Verification items for the finished model (mm, model axes). A direction names the side the tool comes from. Give positions to 0.01 mm unless a question says otherwise; leave off trailing zeros. Loops run counter-clockwise (first coordinate to the right, second up) from the corner with the lowest first, then second, coordinate; pieces in that order, holes last. Notation, with made-up numbers: (17, -12.75) - (59, -12.75) arc R30 ccw to (59, 10.25) - close; hole circle Ø7 at (-33, 62.25). An arc over 180 degrees is marked (long way). Answer in a Markdown table with one row per item.
```python
from build123d import *

# Parameters (mm, degrees)
EXTRUDE_1_DEPTH     = 3
SKETCH_4_W          = 13
SKETCH_4_H          = 8
EXTRUDE_2_DEPTH     = 7
EXTRUDE_6_DEPTH     = 20
CUT_EXTRUDE_3_DEPTH = 34.531337759
EXTRUDE_7_DEPTH     = 16
SKETCH_18_W         = 6.2
SKETCH_18_H         = 1
CUT_EXTRUDE_6_DEPTH = 20
SKETCH_19_R         = 1
CUT_EXTRUDE_7_DEPTH = 3
EXTRUDE_8_DEPTH     = 12
SKETCH_24_W         = 2.5
SKETCH_24_H         = 9.5
CUT_EXTRUDE_8_DEPTH = 20
SKETCH_25_W         = 5
SKETCH_25_H         = 5.2
CUT_EXTRUDE_9_DEPTH = 1


with BuildPart() as part:
    # 草图1 → 凸台-拉伸1 (new body)
    with BuildSketch(Plane(origin=(0, 0, 0), x_dir=(1, 0, 0), z_dir=(0, 1, 0))):
        Polygon((24, 0), (12, 20.784609691), (-12, 20.784609691), (-24, 0), (-12, -20.784609691), (12, -20.784609691), align=None)
    extrude(amount=EXTRUDE_1_DEPTH)

    # 草图4 → 凸台-拉伸2 (add)
    with BuildSketch(Plane(origin=(0, 3, 0), x_dir=(1, 0, 0), z_dir=(0, 1, 0))):
        with Locations((0, -8.746728068)):
            Rectangle(SKETCH_4_W, SKETCH_4_H)
    extrude(amount=EXTRUDE_2_DEPTH)

    # 草图14 → 凸台-拉伸6 (add)
    with BuildSketch(Plane.XY.offset(12.746728068)):
        with BuildLine():
            Line((-6.5, 10), (-6.5, 6.5))
            ThreePointArc((-6.5, 6.5), (0, 5.267826192), (6.5, 6.5))
            Line((6.5, 6.5), (6.5, 10))
            ThreePointArc((6.5, 10), (0, 8.436464997), (-6.5, 10))
        make_face()
    extrude(amount=EXTRUDE_6_DEPTH)

    # 草图15 → 切除-拉伸3 (cut, through all)
    with BuildSketch(Plane.XY.offset(12.746728068)):
        with BuildLine():
            Line((6.5, 10), (-6.5, 10))
            ThreePointArc((-6.5, 10), (0, 8.436464997), (6.5, 10))
        make_face()
    extrude(amount=-CUT_EXTRUDE_3_DEPTH, mode=Mode.SUBTRACT)

    # 草图16 → 凸台-拉伸7 (add)
    with BuildSketch(Plane(origin=(0, 3, 0), x_dir=(1, 0, 0), z_dir=(0, 1, 0))):
        with BuildLine():
            Line((6.5, 13.284609691), (6.5, 11.284609691))
            ThreePointArc((6.5, 11.284609691), (0, 12.623387741), (-6.5, 11.284609691))
            Line((-6.5, 11.284609691), (-6.5, 13.284609691))
            ThreePointArc((-6.5, 13.284609691), (0, 14.747919911), (6.5, 13.284609691))
        make_face()
    extrude(amount=EXTRUDE_7_DEPTH)

    # 草图18 → 切除-拉伸6 (cut, through all)
    with BuildSketch(Plane.XZ):
        Polygon((10.319872981, 13.694675051), (9.453847577, 13.194675051), (12.553847577, 7.825317547), (13.419872981, 8.325317547), align=None)
        Polygon((13.053847577, 6.959292144), (13.919872981, 7.459292144), (17.019872981, 2.08993464), (16.153847577, 1.58993464), align=None)
        with Locations((3.6, -15.284609691)):
            Rectangle(SKETCH_18_W, SKETCH_18_H)
        with Locations((-3.6, -15.284609691)):
            Rectangle(SKETCH_18_W, SKETCH_18_H)
        Polygon((-16.153847577, 1.58993464), (-13.053847577, 6.959292144), (-13.919872981, 7.459292144), (-17.019872981, 2.08993464), align=None)
        Polygon((-12.553847577, 7.825317547), (-13.419872981, 8.325317547), (-10.319872981, 13.694675051), (-9.453847577, 13.194675051), align=None)
    extrude(amount=-CUT_EXTRUDE_6_DEPTH, mode=Mode.SUBTRACT)

    # 草图19 → 切除-拉伸7 (cut)
    with BuildSketch(Plane.XZ):
        with Locations((0, 17.784609691)):
            Circle(SKETCH_19_R)
        with Locations((15.401923789, -8.892304845)):
            Circle(SKETCH_19_R)
        with Locations((-15.401923789, -8.892304845)):
            Circle(SKETCH_19_R)
    extrude(amount=-CUT_EXTRUDE_7_DEPTH, mode=Mode.SUBTRACT)

    # 草图23 → 凸台-拉伸8 (add)
    with BuildSketch(Plane.XY.offset(32.746728068)):
        with BuildLine():
            Line((-9.532090727, 12.079217693), (-9.532090727, 8.042497168))
            ThreePointArc((-9.532090727, 8.042497168), (0, 5.267826192), (9.532090727, 8.042497168))
            Line((9.532090727, 8.042497168), (9.532090727, 12.079217693))
            ThreePointArc((9.532090727, 12.079217693), (0, 8.436464997), (-9.532090727, 12.079217693))
        make_face()
    extrude(amount=EXTRUDE_8_DEPTH)

    # 草图24 → 切除-拉伸8 (cut, through all)
    with BuildSketch(Plane.XZ):
        with Locations((-7.282090727, 38.496728068)):
            Rectangle(SKETCH_24_W, SKETCH_24_H)
        with Locations((7.282090727, 38.496728068)):
            Rectangle(SKETCH_24_W, SKETCH_24_H)
    extrude(amount=-CUT_EXTRUDE_8_DEPTH, mode=Mode.SUBTRACT)

    # 草图25 → 切除-拉伸9 (cut)
    with BuildSketch(Plane.XZ):
        Polygon((-10.532695155, -0.673943767), (-6.029363055, -3.273943767), (-3.529363055, 1.056183252), (-8.032695155, 3.656183252), align=None)
        Polygon((-7.182695155, 5.128426439), (-4.682695155, 9.458553458), (-0.179363055, 6.858553458), (-2.679363055, 2.528426439), align=None)
        Polygon((6.029363055, -3.273943767), (3.529363055, 1.056183252), (8.032695155, 3.656183252), (10.532695155, -0.673943767), align=None)
        Polygon((0.179363055, 6.858553458), (2.679363055, 2.528426439), (7.182695155, 5.128426439), (4.682695155, 9.458553458), align=None)
        with Locations((-3.35, -6.184609691)):
            Rectangle(SKETCH_25_W, SKETCH_25_H)
        with Locations((3.35, -6.184609691)):
            Rectangle(SKETCH_25_W, SKETCH_25_H)
    extrude(amount=-CUT_EXTRUDE_9_DEPTH, mode=Mode.SUBTRACT)


solid = part.part
```
Q1. Thickness scan on line 1 (X direction, y = 10.75, z = 38.5); line 2 (Y direction, x = 18, z = -4); line 3 (X direction, y = 11.75, z = 39). Record the ranges inside material, lowest first.
Completed:
| item | result |
|---|---|
| line 1 | -9.53 to -8.53, 8.53 to 9.53 |
| line 2 | 0 to 3 |
| line 3 | -9.53 to -9.15, 9.15 to 9.53 |
Q2. Sectioned sample at D-D (z = 32). Record the cut outline in (x, y), and give its area (3 significant figures).
Completed:
| item | result |
|---|---|
| outline | (-6.5, 6.5) arc R17.76 ccw to (6.5, 6.5) - (6.5, 10) arc R14.29 cw to (-6.5, 10) - close |
| area | 42.5 mm^2 |
Q3. Draft check along X on faces 1 (the face through (-6.5, 11, -12)), 2 (the face through (14.66, 1.48, -8.22)), 3 (the face through (0, 1, 20.785)). Enter one of: +X half, -X half, draft (parallel to the pull), parting line (faces both ways), or undercut.
Completed:
| item | result |
|---|---|
| face 1 | -X half |
| face 2 | undercut |
| face 3 | draft |
Q4. Sectioned sample at C-C (y = 17.75). Record the cut outline in (x, z), and give its area (3 significant figures).
Completed:
| item | result |
|---|---|
| outline | (-6.5, -13.28) arc R15.17 ccw to (6.5, -13.28) - (6.5, -11.28) arc R16.45 cw to (-6.5, -11.28) - close |
| area | 27.1 mm^2 |
Q5. Go/stop test with flat-tipped pins: P1, Ø4, axis at y = 10.5, z = 11.5, coming from the -X side; P2, Ø2.5, axis at x = 2.5, z = -7, coming from the -Y side; P3, Ø0.5, axis at y = 0.5, z = -5, coming from the -X side. Record where each tip stops, or that it passes through.
Completed:
| item | result |
|---|---|
| P1 | x = -6.5 |
| P2 | y = 1 |
| P3 | x = -21.26 |
Q6. Sectioned sample at B-B (x = 2). Record the cut outline in (y, z), and give its area (3 significant figures).
Completed:
| item | result |
|---|---|
| outline | (0, -20.78) - (3, -20.78) - (3, -15.78) - (0, -15.78) - close; (0, -14.78) - (3, -14.78) - (3, -14.62) - (19, -14.62) - (19, -12.5) - (3, -12.5) - (3, 4.75) - (8.58, 4.75) - (8.58, 44.75) - (5.38, 44.75) - (5.38, 12.75) - (3, 12.75) - (3, 20.78) - (0, 20.78) - (0, 7.91) - (1, 7.91) - (1, 3.71) - (0, 3.71) - (0, -3.58) - (1, -3.58) - (1, -8.78) - (0, -8.78) - close |
| area | 293 mm^2 |
Q7. Sectioned sample at A-A (z = 11). Record the cut outline in (x, y).
Completed:
| item | result |
|---|---|
| outline | (-17.65, 0) - (-11.88, 0) - (-11.88, 3) - (-17.65, 3) - close; (-10.72, 0) - (10.72, 0) - (10.72, 3) - (6.5, 3) - (6.5, 10) arc R14.29 cw to (-6.5, 10) - (-6.5, 3) - (-10.72, 3) - close; (11.88, 0) - (17.65, 0) - (17.65, 3) - (11.88, 3) - close |
Q8. Tool access check on faces 4 (the face through (4.797, 0.493, -1.139)), 5 (the face through (8, 9, 32.747)), 6 (the face through (4, 1, -15.785)), 7 (the face through (0, 6, 4.747)), 8 (the face through (-8, 9, 32.747)). Record the directions out of +Z, -Z, +X, -X, +Y, -Y that give a thin tool (end or side, any length) a straight path to the whole face; none if there is none.
Completed:
| item | result |
|---|---|
| face 4 | -Y |
| face 5 | -Z, +X, +Y, -Y |
| face 6 | +Y, -Y |
| face 7 | +X, -X, +Y |
| face 8 | -Z, -X, +Y, -Y |
